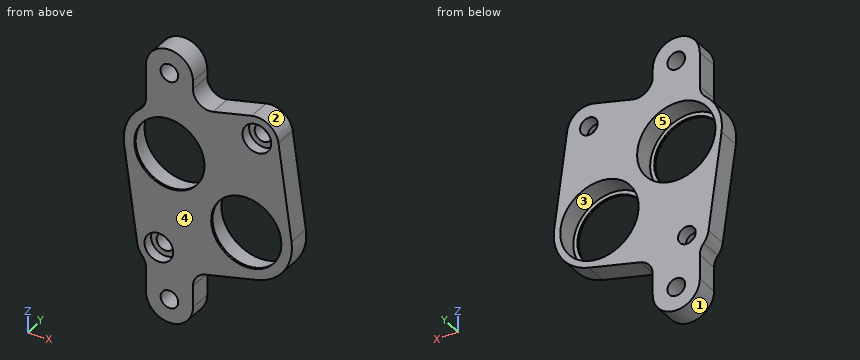
from build123d import *

# Parameters (mm, degrees)
SKETCH1_R           = 7.626999986
SKETCH1_R_2         = 1.7145
BOSS_EXTRUDE1_DEPTH = 4.000000128
BOSS_EXTRUDE2_START = 0.396875
SKETCH2_R           = 6.833249986
BOSS_EXTRUDE2_DEPTH = 0.396875
SKETCH3_R           = 2.794
CUT_EXTRUDE1_DEPTH  = 2.032
SKETCH6_R           = 1.7145
BOSS_EXTRUDE5_DEPTH = 4.396875128
FILLET1_R           = 3.175


with BuildPart() as part:
    # Sketch1 → Boss-Extrude1 (new body)
    with BuildSketch(Plane(origin=(0, 0, 0), x_dir=(-1, 0, 0), z_dir=(0, -1, 0))):
        with BuildLine():
            Line((-21.238527151, -9.504108586), (-23.776738447, 8.97469386))
            ThreePointArc((-23.776738447, 8.97469386), (-22.317172851, 15.191935329), (-17.068206789, 18.829623948))
            Line((-17.068206789, 18.829623948), (1.054165054, 23.244178876))
            ThreePointArc((1.054165054, 23.244178876), (4.455202947, 22.62752212), (6.276027151, 19.689508586))
            Line((6.276027151, 19.689508586), (8.814238447, 1.21070614))
            ThreePointArc((8.814238447, 1.21070614), (7.354672851, -5.006535329), (2.105706789, -8.644223948))
            Line((2.105706789, -8.644223948), (-16.016665054, -13.058778876))
            ThreePointArc((-16.016665054, -13.058778876), (-19.417702947, -12.44212212), (-21.238527151, -9.504108586))
        make_face()
        with Locations(Location((-14.9625, 10.1854, 0), (0, 0, 90))):
            Circle(SKETCH1_R, mode=Mode.SUBTRACT)
        with Locations(Location((0, 0, 0), (0, 0, 90))):
            Circle(SKETCH1_R, mode=Mode.SUBTRACT)
        with Locations(Location((2.061103297, 19.110555087, 0), (0, 0, 90))):
            Circle(SKETCH1_R_2, mode=Mode.SUBTRACT)
        with Locations(Location((-17.023603297, -8.925155087, 0), (0, 0, 90))):
            Circle(SKETCH1_R_2, mode=Mode.SUBTRACT)
    extrude(amount=-BOSS_EXTRUDE1_DEPTH)

    # Sketch2 → Boss-Extrude2 (add)
    with BuildSketch(Plane.XZ.offset(BOSS_EXTRUDE2_START)):
        with BuildLine():
            Line((16.016665054, 13.058778876), (-2.105706789, 8.644223948))
            ThreePointArc((-2.105706789, 8.644223948), (-7.354672851, 5.006535329), (-8.814238447, -1.21070614))
            Line((-8.814238447, -1.21070614), (-6.276027151, -19.689508586))
            ThreePointArc((-6.276027151, -19.689508586), (-4.455202947, -22.62752212), (-1.054165054, -23.244178876))
            Line((-1.054165054, -23.244178876), (17.068206789, -18.829623948))
            ThreePointArc((17.068206789, -18.829623948), (22.317172851, -15.191935329), (23.776738447, -8.97469386))
            Line((23.776738447, -8.97469386), (21.238527151, 9.504108586))
            ThreePointArc((21.238527151, 9.504108586), (19.417702947, 12.44212212), (16.016665054, 13.058778876))
        make_face()
        with Locations(Location((14.9625, -10.1854, 0), (0, 0, 270))):
            Circle(SKETCH2_R, mode=Mode.SUBTRACT)
        with Locations(Location((0, 0, 0), (0, 0, 270))):
            Circle(SKETCH2_R, mode=Mode.SUBTRACT)
    extrude(amount=-BOSS_EXTRUDE2_DEPTH)

    # Sketch3 → Cut-Extrude1 (cut)
    with BuildSketch(Plane.XZ.offset(0.396875)):
        with Locations(Location((17.023603297, 8.925155087, 0), (0, 0, 270))):
            Circle(SKETCH3_R)
        with Locations(Location((-2.061103297, -19.110555087, 0), (0, 0, 270))):
            Circle(SKETCH3_R)
    extrude(amount=-CUT_EXTRUDE1_DEPTH, mode=Mode.SUBTRACT)

    # Sketch6 → Boss-Extrude5 (add)
    # profile 1 of 2: a face of its own
    with BuildSketch(Plane.XZ.offset(0.396875)):
        with BuildLine():
            Line((-4.580991155, 7.626999986), (-4.580991155, 15.875))
            ThreePointArc((-4.580991155, 15.875), (0, 20.455991155), (4.580991155, 15.875))
            Line((4.580991155, 15.875), (4.580991155, 10.273083328))
            Line((4.580991155, 10.273083328), (-2.105706789, 8.644223948))
            ThreePointArc((-2.105706789, 8.644223948), (-3.381814379, 8.229212614), (-4.580991155, 7.626999986))
        make_face()
        with Locations(Location((0, 15.875, 0), (0, 0, 270))):
            Circle(SKETCH6_R, mode=Mode.SUBTRACT)
    # profile 2 of 2: a face of its own
    with BuildSketch(Plane.XZ.offset(0.396875)):
        with BuildLine():
            Line((-4.580991155, -22.538518831), (-4.580991155, -28.575))
            ThreePointArc((-4.580991155, -28.575), (0, -33.155991155), (4.580991155, -28.575))
            Line((4.580991155, -28.575), (4.580991155, -21.87147188))
            Line((4.580991155, -21.87147188), (-1.054165054, -23.244178876))
            ThreePointArc((-1.054165054, -23.244178876), (-2.89581472, -23.282368493), (-4.580991155, -22.538518831))
        make_face()
        with Locations(Location((0, -28.575, 0), (0, 0, 270))):
            Circle(SKETCH6_R, mode=Mode.SUBTRACT)
    extrude(amount=-BOSS_EXTRUDE5_DEPTH)

    # Fillet1
    fillet1_edges = [part.edges().sort_by_distance(p)[0] for p in [
        (4.580991155, 1.801562564, 10.273083328),
        (-4.580991155, 1.801562564, 7.626999986),
        (4.580991155, 1.801562564, -21.87147188),
        (-4.580991155, 1.801562564, -22.538518831),
    ]]
    fillet(fillet1_edges, radius=FILLET1_R)


solid = part.part
Part model, mm, in its own coordinate system. Face numbers are marked on the shaded views. A direction names the side the tool comes from. Give positions to 0.01 mm unless a question says otherwise; leave off trailing zeros. Loops run counter-clockwise (first coordinate to the right, second up) from the corner with the lowest first, then second, coordinate; pieces in that order, holes last. Notation, with made-up numbers: (29, 78.5) -> (83, 78.5) arc R20 cw to (83, 103.5) -> close; hole circle Ø10 at (-34.75, 33.25). An arc over 180 degrees is marked (long way). Write each question's results on one line, items separated by ' | '. Start each with the question number.
Q1. Band-saw the part on A-A on z = -14. List the corners of the cut face in (x, y), plus the area to 3 significant figures.
Q2. Pin check, flat tips, straight feed: P1, Ø17, axis at x = 1, z = 0.5, coming from the +Y side; P2, Ø1, axis at y = 3, z = -3, coming from the -X side; P3, Ø1, axis at x = 4.5, y = 2.5, coming from the -Z side; P4, Ø1.3, axis at y = 0.5, z = -25.5, coming from the +X side. Stop position of each tip, or through.
Q3. Band-saw the part on C-C on z = -26. List the corners of the cut face in (x, y), plus the area to 3 significant figures.
Q4. Which spindle directions (+Z, -Z, +X, -X, +Y, -Y) get a long thin tool onto all of the face, cutting with end or side? Do the marked faces 4 and 5. Say none if no direction does.
Q5. Wall check: L1, parallel to X at y = 2.2, z = 16; L2, parallel to X at y = 1.7, z = -6; L3, parallel to Z at x = -0.5, y = 3.1. Give the ranges that are in metal, low to high.
Q6. Pull direction Z, two halves, no side cores. Call the marked faces 1, 2 and 3: +Z half, -Z half, draft (parallel to the pull), parting line (faces both ways), or undercut.
Q7. Band-saw the part on B-B on x = 20.5. List the corners of the cut face in (y, z), plus the area to 3 significant figures.
Results are:
1) outline: (-7.06, -0.4) -> (9.29, -0.4) -> (9.29, 0) -> (8.36, 0) -> (8.36, 4) -> (-7.06, 4) -> close; (20.63, -0.4) -> (23, -0.4) -> (23, 4) -> (21.57, 4) -> (21.57, 0) -> (20.63, 0) -> close | area: 74.8 mm²
2) P1: stops at y = 4 | P2: stops at x = -8.64 | P3: stops at z = -30.81 | P4: stops at x = 4.58
3) outline: (-4.58, -0.4) -> (4.58, -0.4) -> (4.58, 4) -> (-4.58, 4) -> close | area: 40.3 mm²
4) face 4: +Z, -Z, +X, -X, -Y | face 5: +Y
5) L1: x = -4.58 to -1.71, 1.71 to 4.58 | L2: x = -8.16 to -4.71, 4.71 to 8.59, 21.34 to 23.37 | L3: z = -33.13 to -30.21, -26.94 to -19.82, -18.4 to -7.61, 7.61 to 14.24, 17.51 to 20.43
6) face 1: -Z half | face 2: +Z half | face 3: undercut
7) outline: (-0.4, -17.15) -> (4, -17.15) -> (4, -15.43) -> (0, -15.43) -> (0, -14.19) -> (-0.4, -14.19) -> close; (-0.4, -6.18) -> (0, -6.18) -> (0, -4.94) -> (4, -4.94) -> (4, 11.38) -> (-0.4, 11.38) -> close | area: 80.3 mm²
